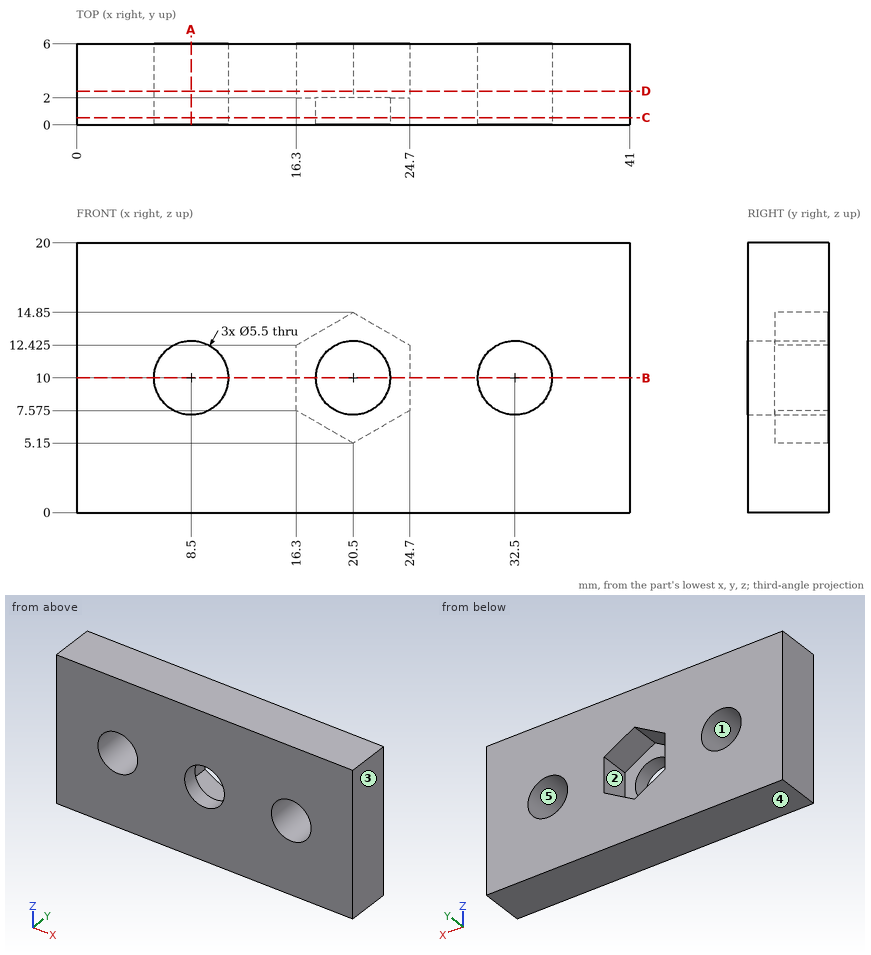
Verification items for this drawing (mm, ordinates from the low corner). A direction names the side the tool comes from. Round coordinates to 2 decimals unless told otherwise and drop trailing zeros. Write each loop counter-clockwise with the first axis right and the second up, starting at its lowest first coordinate (ties: lowest second). Pieces come first, ordered by that corner, then holes. Notation, with made-up numbers: M -34.5,-36.5 L -15.5,-36.5 A36 ccw -15.5,0.5 Z; hole C 48,-3.5 d8. An arc over 180 degrees is marked long. Write item = value, one per line. Start each with the question number.
1. Scan lines: line 1 (X direction, y = 2.7, z = 10); line 2 (X direction, y = 1.05, z = 10); line 3 (Z direction, x = 8.5, y = 4.7). Record each from-to range of solid material in increasing order. Write a range as [from, to].
2. Section check C-C, the plane y = 0.55. Record the cut outline in (x, z), then the cut area to 3 significant figures.
3. Release check for a two-part mould opening along X. For the marked faces 3, 4 and 5 record: pulls with the +X half, pulls with the -X half, needs draft (parallel to the pull), parting line crosses it, or undercut.
4. Section check D-D, the plane y = 2.5. State how many separate pieces and enclosed holes the cut face has, then the cut area to 3 significant figures.
5. Section check B-B, the plane z = 10. Record the cut outline in (x, y), then the cut area to 3 significant figures.
6. Tool access check on the marked faces 1 and 2. Record the directions out of +Z, -Z, +X, -X, +Y, -Y that give a thin tool (end or side, any length) a straight path to the whole face; none if there is none.
7. Section check A-A, the plane x = 8.5. Record the cut outline in (y, z).
8. Gauge pin test, flat end, axial feed: pin 1 (5 mm diameter, centred on x = 20.5, z = 10, fed in from -Y). Record the tip position at first contact, or that the pin passes through.
Results found:
q1.line_1 = [0, 5.75], [11.25, 16.3], [24.7, 29.75], [35.25, 41]
q1.line_2 = [0, 5.75], [11.25, 17.75], [23.25, 29.75], [35.25, 41]
q1.line_3 = [0, 7.25], [12.75, 20]
q2.outline = M 0,0 L 41,0 L 41,20 L 0,20 Z; hole C 8.5,10 d5.5; hole C 20.5,10 d5.5; hole C 32.5,10 d5.5
q2.area = 749 mm^2
q3.face_3 = pulls with the +X half
q3.face_4 = needs draft
q3.face_5 = undercut
q4.separate_pieces = 1
q4.enclosed_holes = 3
q4.area = 711 mm^2
q5.outline = M 0,0 L 5.75,0 L 5.75,6 L 0,6 Z; M 11.25,0 L 17.75,0 L 17.75,2 L 16.3,2 L 16.3,6 L 11.25,6 Z; M 23.25,0 L 29.75,0 L 29.75,6 L 24.7,6 L 24.7,2 L 23.25,2 Z; M 35.25,0 L 41,0 L 41,6 L 35.25,6 Z
q5.area = 135 mm^2
q6.face_1 = +Y, -Y
q6.face_2 = +Y
q7.outline = M 0,0 L 6,0 L 6,7.25 L 0,7.25 Z; M 0,12.75 L 6,12.75 L 6,20 L 0,20 Z
q8.pin_1 = through
